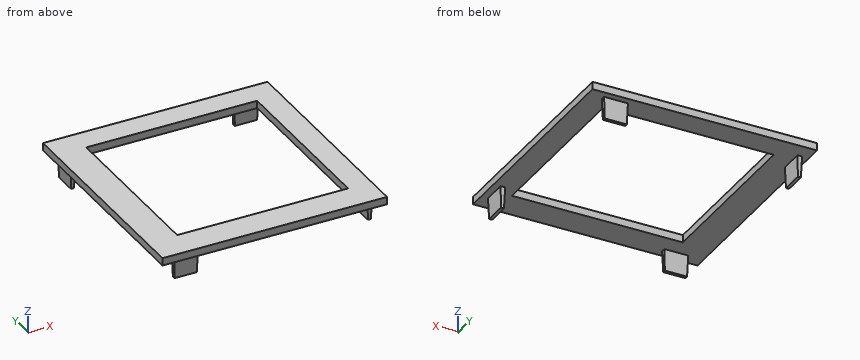
```python
from build123d import *

# Parameters (mm, degrees)
F0_W     = 59.5
F0_H     = 59.5
F0_W_2   = 45.3
F0_H_2   = 45.3
F1_DEPTH = 2
F2_W     = 1.2
F2_H     = 6.3
F2_W_2   = 6.3
F2_H_2   = 1.2
F3_DEPTH = 5.7
F3_TAPER = 2


# Not quite as in the source:
# - a feature names something its author has since deleted; it is built from what else it names


with BuildPart() as f1:
    # F0 (on Top) → F1 (new body)
    with BuildSketch(Plane.XY):
        Rectangle(F0_W, F0_H)
        with Locations((0.8918590039, 0.6)):
            Rectangle(F0_W_2, F0_H_2, mode=Mode.SUBTRACT)
    extrude(amount=F1_DEPTH)

    # F2 (on face) → F3 (join)
    with BuildSketch(Plane(origin=(0, 0, 0), x_dir=(1, 0, 0), z_dir=(0, 0, -1))):
        with Locations((27.3418590039, 22.55)):
            Rectangle(F2_W, F2_H)
        with Locations((22.55, -27.3418590039)):
            Rectangle(F2_W_2, F2_H_2)
        with Locations((-27.3418590039, -22.55)):
            Rectangle(F2_W, F2_H)
        with Locations((-22.55, 27.3418590039)):
            Rectangle(F2_W_2, F2_H_2)
    extrude(amount=F3_DEPTH, taper=F3_TAPER)


solid = f1.part
```
Check sheet for the modelled part. Datum: model origin and axes. Units: mm. Give positions to 0.01 mm unless a question says otherwise; leave off trailing zeros. Write each loop counter-clockwise with the first axis right and the second up, starting at its lowest first coordinate (ties: lowest second). Pieces come first, ordered by that corner, then holes.
Item 1: Cross-section at B-B (x = -13.5). Enter the section's corners in (y, z), and give its area (3 significant figures).
Item 2: Cross-section at D-D (z = -3). Count the separate pieces of the cut face and the enclosed holes in it, and give its area (3 significant figures).
Item 3: Cross-section at A-A (y = -8). Enter the section's corners in (x, z).
Item 4: Scan lines: L1, parallel to Z at x = -25.5, y = -7; L2, parallel to Y at x = 19, z = 1.25; L3, parallel to X at y = -21, z = -2.5. Record each from-to range of solid material in increasing order.
Item 5: Cross-section at C-C (z = 0.75). Enter the section's corners in (x, y).
Report:
1. outline: (-29.75, 0) - (-22.05, 0) - (-22.05, 2) - (-29.75, 2) - close; (23.25, 0) - (29.75, 0) - (29.75, 2) - (23.25, 2) - close
1. area: 28.4 mm2
2. separate pieces: 4
2. enclosed holes: 0
2. area: 24.1 mm2
3. outline: (-29.75, 0) - (-21.76, 0) - (-21.76, 2) - (-29.75, 2) - close; (23.54, 0) - (29.75, 0) - (29.75, 2) - (23.54, 2) - close
4. L1: z = 0 to 2
4. L2: y = -29.75 to -22.05, 23.25 to 29.75
4. L3: x = 26.83 to 27.85
5. outline: (-29.75, -29.75) - (29.75, -29.75) - (29.75, 29.75) - (-29.75, 29.75) - close; hole (-21.76, -22.05) - (23.54, -22.05) - (23.54, 23.25) - (-21.76, 23.25) - close
